Source: CAD feature listing. Evaluate the final solid. Frame: model axes, mm. A direction names the side the tool comes from. Coordinates: 2 decimals unless noted, no trailing zeros. Loops run counter-clockwise (first coordinate to the right, second up) from the corner with the lowest first, then second, coordinate; pieces in that order, holes last. Notation, with made-up numbers: M 68,51 L 126,51 A19 ccw 126,72 Z; hole C -23.75,54.25 d7. An arc over 180 degrees is marked long. One line per question, with ' | ' between items. Start each with the question number.
1. Pin query (flat end, axial travel): P1, Ø1.5, axis at x = -19, y = -8, coming from the -Z side; P2, Ø2, axis at x = -58, z = -1.5, coming from the -Y side; P3, Ø8, axis at x = -19, y = 0, coming from the -Z side. Return the tip coordinate at first contact, or that it passes through.
2. Access query for faces 1 (the flat face through (-96, 2, 5)), 2 (the cylindrical face through (-108.353, -1.802, -5.723)), 3 (the flat face through (-120, 0, 0)), 4 (the cylindrical face through (-21.5, 0.1, 0.1)), 5 (the cylindrical face through (-15.8, 7.81, 1.73)). Directions: +Z, -Z, +X, -X, +Y, -Y. A direction counts if a zero-diameter tool reaches every point of the face in a straight line with its end or side. Return the directions, or none.
3. Section query B-B, the plane z = 0. Output: boundary loops of the cut face in (x, y), and give its area (3 significant figures).
4. Section query C-C, the plane x = -102. Output: boundary loops of the cut face in (y, z).
5. Mould query, pull axis X, two halves, no side actions, for faces 6 (the flat face through (0, 0, 0)), 7 (the flat face through (-98, -4, 4)), 8 (the cylindrical face through (-63.6, -11.4, 1.5)). Classes: pulls with the +X half, pulls with the -X half, needs draft (parallel to the pull), parting line crosses it, or undercut.
6. Ray query, probe 1 along X at (y, z) = (0, 0.25); probe 2 along Y at (x, z) = (-19, -0.25); probe 3 along X at (y, z) = (1.5, 5.5). Return the intervals inside material, ascending.
7. Section query A-A, the plane y = 0. Output: boundary loops of the cut face in (x, z).
8. Section query D-D, the plane x = -19. Output: boundary loops of the cut face in (y, z), and give its area (3 significant figures).
```python
from build123d import *

# Parameters (mm, degrees)
SKETCH3_R          = 2.5
CUT_EXTRUDE1_DEPTH = 10
CHAMFER1_SIZE      = 2
CHAMFER2_SIZE      = 1


with BuildPart() as part:
    # Sketch2 → Revolve1 (revolve)
    with BuildSketch(Plane.XY, mode=Mode.PRIVATE) as revolve1_sk:
        Polygon((0, 0), (-30, 0), (-32, 0), (-96, 0), (-98, 0), (-120, 0), (-120, 6), (-98, 6), (-98, 5), (-96, 5), (-96, 11.5), (-32, 11.5), (-32, 7), (-30, 7), (-30, 8), (0, 8), align=None)
    revolve(revolve1_sk.sketch.rotate(Axis((0, 0, 0), (-1, 0, 0)), 90), axis=Axis((0, 0, 0), (-1, 0, 0)))

    # Sketch3 → Cut-Extrude1 (cut, symmetric)
    with BuildSketch(Plane.XY):
        with Locations((-19, 0)):
            Circle(SKETCH3_R)
    extrude(amount=CUT_EXTRUDE1_DEPTH, both=True, mode=Mode.SUBTRACT)

    # Chamfer1
    chamfer1_edges = [part.edges().sort_by_distance(p)[0] for p in [
        (0, 0, 8),
    ]]
    chamfer(chamfer1_edges, length=CHAMFER1_SIZE)

    # Chamfer2
    chamfer2_edges = [part.edges().sort_by_distance(p)[0] for p in [
        (-120, 0, 6),
    ]]
    chamfer(chamfer2_edges, length=CHAMFER2_SIZE)


solid = part.part
```
Taken from the geometry:
1) P1: z = -3.38 | P2: y = -11.49 | P3: z = -8
2) face 1: none | face 2: -X | face 3: +Z, -Z, -X, +Y, -Y | face 4: +Z, -Z | face 5: +X
3) outline: M -120,-5 L -119,-6 L -98,-6 L -98,-5 L -96,-5 L -96,-11.5 L -32,-11.5 L -32,-7 L -30,-7 L -30,-8 L -2,-8 L 0,-6 L 0,6 L -2,8 L -30,8 L -30,7 L -32,7 L -32,11.5 L -96,11.5 L -96,5 L -98,5 L -98,6 L -119,6 L -120,5 Z; hole C -19,0 d5 | area: 2,240 mm^2
4) outline: C 0,0 d12
5) face 6: pulls with the +X half | face 7: undercut | face 8: needs draft
6) probe 1: -120 to -21.5, -16.5 to 0 | probe 2: -8 to -2.5, 2.5 to 8 | probe 3: -119.3 to -98, -96 to -21, -17 to 0
7) outline: M -120,-5 L -119,-6 L -98,-6 L -98,-5 L -96,-5 L -96,-11.5 L -32,-11.5 L -32,-7 L -30,-7 L -30,-8 L -21.5,-8 L -21.5,8 L -30,8 L -30,7 L -32,7 L -32,11.5 L -96,11.5 L -96,5 L -98,5 L -98,6 L -119,6 L -120,5 Z; M -16.5,-8 L -2,-8 L 0,-6 L 0,6 L -2,8 L -16.5,8 Z
8) outline: M -2.5,-7.6 L -2.5,7.6 A8 ccw Z; M 2.5,-7.6 A8 ccw 2.5,7.6 Z | area: 122 mm^2
